Verification items for the finished model (mm, model axes). Face numbers are marked on the shaded views. A direction names the side the tool comes from. Give positions to 0.01 mm unless a question says otherwise; leave off trailing zeros. Order: outer loops, then holes, each group sorted by start corner. A loop starts at its lowest first (then second) coordinate and runs counter-clockwise, first axis right, second up.
(1) Mould release check, pull along X, two halves, no side actions. Record for the marked faces 4, 5 and 6: pulls with the +X half, pulls with the -X half, needs draft (parallel to the pull), parting line crosses it, or undercut.
(2) Scan lines: L1, parallel to Z at x = 28, y = -8.5; L2, parallel to X at y = 6, z = 10.5; L3, parallel to X at y = -13, z = 34. Record each from-to range of solid material in increasing order.
(3) Gauge pin test, flat ends, axial feed: pin 1 (15 mm diameter, centred on y = -6, z = 21.5, fed in from +X); pin 2 (3 mm diameter, centred on x = 18, y = 8, fed in from +Z); pin 3 (2 mm diameter, centred on x = -6.5, y = -6, fed in from +Z). Record the tip position at first contact, or that the pin passes through.
(4) Access from +Z, -Z, +X, -X, +Y, -Y to the whole of each face (thin tool, end or side, straight path). Record for the marked faces 1, 2 and 3.
(5) Sectioned sample at B-B on x = -25.5. Record the cut outline in (y, z), plus the area to 3 significant figures.
(6) Sectioned sample at C-C on z = 21. Record the cut outline in (x, y), plus the area to 3 significant figures.
```python
from build123d import *

# Parameters (mm, degrees)
F0_W     = 80
F0_H     = 30
F1_DEPTH = 10
F2_SIZE  = 9.99999
F4_DEPTH = 15
F5_DEPTH = 15


# Not quite as in the source:
# - a fillet or chamfer is up to 0.001 mm smaller than in the source, because OpenCascade refuses the exact size


with BuildPart() as f1:
    # F0 (on Top) → F1 (new body)
    with BuildSketch(Plane.XY):
        Rectangle(F0_W, F0_H)
    extrude(amount=F1_DEPTH)

    # F2 (size 10 in the source; OpenCascade refuses exactly that, so slightly less here)
    f2_edges = [f1.edges().sort_by_distance(p)[0] for p in [
        (-40, 0, 10),
        (40, 0, 10),
    ]]
    chamfer(f2_edges, length=F2_SIZE)

    # F3 (on Front) → F4 (join)
    with BuildSketch(Plane.XZ):
        with BuildLine():
            Line((-15, 10), (15, 10))
            Line((15, 10), (15, 40))
            ThreePointArc((15, 40), (0, 25), (-15, 40))
            Line((-15, 40), (-15, 10))
        make_face()
    extrude(amount=F4_DEPTH)

    # F5 (add): a face of the model
    f5_faces = [f1.faces().sort_by_distance(p)[0] for p in [
        (0, 0, 19.4171231702),
    ]]
    extrude(f5_faces, amount=F5_DEPTH)


solid = f1.part
```
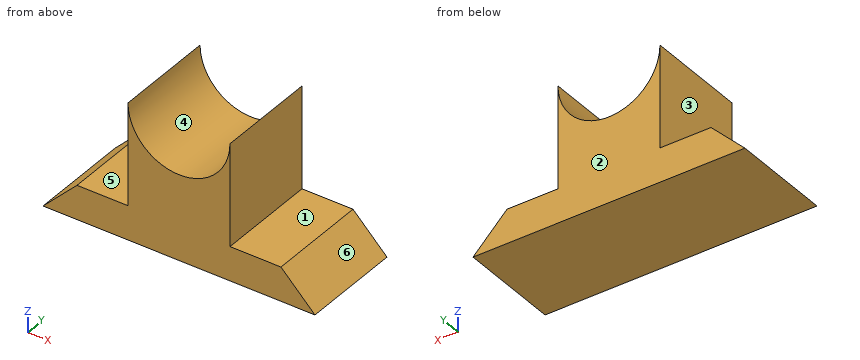
Ans:
1. face 4: undercut
1. face 5: needs draft
1. face 6: pulls with the +X half
2. L1: z = 0 to 10
2. L2: x = -15 to 15
2. L3: x = -15 to -13.75, 13.75 to 15
3. pin 1: stops at x = 15
3. pin 2: stops at z = 10
3. pin 3: stops at z = 27.01
4. face 1: +Z, +X, +Y, -Y
4. face 2: +Z, -Z, +X, -X, +Y
4. face 3: +Z, -X, +Y, -Y
5. outline: (-15, 0) - (15, 0) - (15, 10) - (-15, 10) - close
5. area: 300 mm2
6. outline: (-15, -15) - (15, -15) - (15, 15) - (-15, 15) - close
6. area: 900 mm2
